Read the model definition and answer for the solid it produces. Units are mm, in the model's axes. A direction names the side the tool comes from. Coordinates: 2 decimals unless noted, no trailing zeros. Order: outer loops, then holes, each group sorted by start corner. A loop starts at its lowest first (then second) coordinate and runs counter-clockwise, first axis right, second up. Notation, with made-up numbers: M 17.25,31.5 L 47.25,31.5 A33 cw 47.25,63.5 Z; hole C 29.25,-38.5 d1. An arc over 180 degrees is marked long. Put each result on its own line as item: value.
Autodesk Fusion 360 part; units mm, degrees
sketch "Sketch1" plane through (0, 0, 0) normal (0, 0, 1) x (1, 0, 0)
  circle A0 centre (17.385, 5) radius 20.5
  line L0 (0, 8.75) -> (0, 8.6219)
  line L1 (-0.615, 1.25) -> (0, 1.3781) construction
  line L2 (0, 8.6219) -> (0, 8.75)
  line L3 (0, 1.25) -> (-0.615, 1.25)
  line L4 (-0.615, 1) -> (-0.615, 9)
  line L5 (35.385, 9) -> (35.385, 1)
  line L6 (-0.615, 9) -> (2.1514, 9)
  line L7 (32.6186, 9) -> (35.385, 9)
  line L8 (2.1514, 1) -> (-0.615, 1)
  arc A1 (2.1514, 1) -> (32.6186, 1) centre (17.385, 5) ccw
  arc A2 (32.6186, 9) -> (2.1514, 9) centre (17.385, 5) ccw
  line L9 (32.6186, 1) -> (35.385, 1)
  point P0 (17.385, 5)
  point P1 (17.385, 5)
  point P2 (17.385, 5)
  dimension "d4" = 41
  dimension "d11" = 36
  dimension "d12" = 8
  dimension "d13" = 31.5
extrude "Extrude1" add sketch "Sketch1" along normal blind 4
Q1. Find section B-B on x = 31. Write down the section's boundary in (y, z).
Answers below:
outline: M -10.33,0 L -2.92,0 L -2.92,4 L -10.33,4 Z; M 12.92,0 L 20.33,0 L 20.33,4 L 12.92,4 Z
Q2. Find section A-A on y = 5. Write down the section's boundary in (x, z) (3 decimals).
Answers below:
outline: M -3.115,0 L -0.615,0 L -0.615,4 L -3.115,4 Z; M 35.385,0 L 37.885,0 L 37.885,4 L 35.385,4 Z
Q3. Given pin 1 (1 mm diameter, centred on x = 15, z = 3, fed in from -Y); pin 2 (2 mm diameter, centred on x = 8, z = 1.5, fed in from +Y); pin 3 (8 mm diameter, centred on x = 13.5, y = 13.5, fed in from -Z); pin 4 (0.8 mm diameter, centred on x = 1, z = 1.5, fed in from +Y), each flat-ended and moving along its own axis, determine where each tip first touches the part or whether it passes through.
Answers below:
pin 1: stops at y = -15.41
pin 2: stops at y = 23.71
pin 3: passes through
pin 4: stops at y = 17.83
Q4. Find section D-D on y = -12. Write down the section's boundary in (x, z).
Answers below:
outline: M 5.93,0 L 28.84,0 L 28.84,4 L 5.93,4 Z
Q5. Consider line 1 along Y through (x, z) = (17.5, 3.15); line 2 along X through (y, z) = (5.5, 1.65) (3 decimals); line 3 along Y through (x, z) = (7, 3). Determine where each line is inside the solid, lowest interval first.
Answers below:
line 1: y = -15.5 to -10.75, 20.75 to 25.5
line 2: x = -3.109 to -0.615, 35.385 to 37.879
line 3: y = -12.67 to -6.84, 16.84 to 22.67
Q6. A tool of negligible diameter and unlimited length cuts with its end or side. For faces 1 (the face through (28, -7, 4)), 2 (the face through (17.095, 20.747, 1.972)), from which of +Z, -Z, +X, -X, +Y, -Y can it reach the whole face along a straight path? Write none if from no direction.
Answers below:
face 1: +Z, +X, -X, +Y, -Y
face 2: +Z, -Z
Q7. For a pull along X with two mould halves and no side action, classify faces 3 (the face through (34, 1, 2)), 4 (the face through (28, -7, 0)), 5 (the face through (2.276, -8.855, 1.972)) as +X half, -X half, draft (parallel to the pull), parting line (faces both ways), or undercut.
Answers below:
face 3: undercut
face 4: draft
face 5: parting line
Q8. Find section C-C on z = 2.05. Write down the section's boundary in (x, y) (3 decimals), plus the area to 3 significant figures.
Answers below:
outline: C 17.385,5 d41; hole M -0.615,1 L 2.151,1 A15.75 ccw 32.619,1 L 35.385,1 L 35.385,9 L 32.619,9 A15.75 ccw 2.151,9 L -0.615,9 Z
area: 502 mm^2
